Input: part model. Units: mm. Frame: model coordinates. A direction names the side the tool comes from. Give positions to 0.01 mm unless a question says otherwise; leave off trailing zeros. Loops run counter-clockwise (first coordinate to the right, second up) from the corner with the lowest first, then second, coordinate; pieces in that order, holes last. Notation, with made-up numbers: (-19.5, 82.5) -> (-13.5, 82.5) arc R22 ccw to (-13.5, 106.5) -> close; hole circle Ø7 at (56.25, 15.25). An arc over 180 degrees is marked (long way). Use CSV: the item, a comma, the result in double quotes.
```python
from build123d import *

# Parameters (mm, degrees)
SKETCH_1_R               = 3
EXTRUDE_1_DEPTH          = 180
SKETCH_2_R               = 8
EXTRUDE_2_DEPTH          = 2
EXTRUDE_START            = -178
SKETCH_2_2_R             = 8
EXTRUDE_3_DEPTH          = 2
EXTRUDE_START_2          = -2
SKETCH_1_2_R             = 3
EXTRUDE_4_DEPTH          = 2
EXTRUDE_START_3          = 180
SKETCH_1_3_R             = 3
EXTRUDE_5_DEPTH          = 2
EXTRUDE_START_4          = 4
SKETCH_2_3_R             = 8
EXTRUDE_6_DEPTH          = 2
EXTRUDE_START_5          = -182
SKETCH_2_4_R             = 8
EXTRUDE_7_DEPTH          = 2
EXTRUDE_START_6          = -64
SKETCH_3_R               = 5
EXTRUDE_10_DEPTH         = 60
CUT_EXTRUDE_1_DEPTH      = 185.347497949
CUT_EXTRUDE_1_DEPTH_BACK = 185.347497949
SKETCH_4_W               = 115.941163498
SKETCH_4_H               = 45.19740272


with BuildPart() as part:
    # 草图1 → 凸台-拉伸1 (new body)
    with BuildSketch(Plane.XY):
        with Locations(Location((0, 0, 0), (0, 0, 180))):
            Circle(SKETCH_1_R)
    extrude(amount=EXTRUDE_1_DEPTH)

    # 草图2 → 凸台-拉伸2 (add)
    with BuildSketch(Plane.XY.offset(180)):
        Circle(SKETCH_2_R)
    extrude(amount=-EXTRUDE_2_DEPTH)

    # 草图2<2> → 凸台-拉伸3 (add)
    with BuildSketch(Plane.XY.offset(180).offset(EXTRUDE_START)):
        Circle(SKETCH_2_2_R)
    extrude(amount=-EXTRUDE_3_DEPTH)

    # 草图1<2> → 凸台-拉伸4 (add)
    with BuildSketch(Plane.XY.offset(EXTRUDE_START_2)):
        with Locations(Location((0, 0, 0), (0, 0, 180))):
            Circle(SKETCH_1_2_R)
    extrude(amount=EXTRUDE_4_DEPTH)

    # 草图1<3> → 凸台-拉伸5 (add)
    with BuildSketch(Plane.XY.offset(EXTRUDE_START_3)):
        with Locations(Location((0, 0, 0), (0, 0, 180))):
            Circle(SKETCH_1_3_R)
    extrude(amount=EXTRUDE_5_DEPTH)

    # 草图2<3> → 凸台-拉伸6 (add)
    with BuildSketch(Plane.XY.offset(180).offset(EXTRUDE_START_4)):
        Circle(SKETCH_2_3_R)
    extrude(amount=-EXTRUDE_6_DEPTH)

    # 草图2<4> → 凸台-拉伸7 (add)
    with BuildSketch(Plane.XY.offset(180).offset(EXTRUDE_START_5)):
        Circle(SKETCH_2_4_R)
    extrude(amount=-EXTRUDE_7_DEPTH)

    # 草图3 → 凸台-拉伸10 (add)
    with BuildSketch(Plane.XY.offset(184).offset(EXTRUDE_START_6)):
        Circle(SKETCH_3_R)
    extrude(amount=-EXTRUDE_10_DEPTH)

    # 草图4 → 切除-拉伸1 (cut, two sides: drawn at the far end of the back side and taken through both)
    with BuildSketch(Plane(origin=(0, 0, 0), x_dir=(0, 0, -1), z_dir=(1, 0, 0)).offset(-CUT_EXTRUDE_1_DEPTH_BACK)):
        with Locations((-38.8417804, 0.262013929)):
            Rectangle(SKETCH_4_W, SKETCH_4_H)
    extrude(amount=CUT_EXTRUDE_1_DEPTH + CUT_EXTRUDE_1_DEPTH_BACK, mode=Mode.SUBTRACT)


solid = part.part
```
1) Contact query for flat-ended pins moving along their axis: pin 1 (4 mm diameter, centred on x = 0.5, z = 127.5, fed in from -Y); pin 2 (3 mm diameter, centred on x = -5.5, z = 145, fed in from -Y); pin 3 (2 mm diameter, centred on x = -1.5, z = 113, fed in from +Y); pin 4 (6 mm diameter, centred on x = 1.5, z = 122, fed in from -Y). Output: stop coordinate, or through.
From the geometry:
pin 1,"stops at y = -3"
pin 2,"passes through"
pin 3,"stops at y = 4.97"
pin 4,"stops at y = -5"
2) Section query C-C (x = -3.75). Return loops of the section in (y, z).
From the geometry:
outline,"(-7.07, 178) -> (7.07, 178) -> (7.07, 180) -> (-7.07, 180) -> close; (-7.07, 182) -> (7.07, 182) -> (7.07, 184) -> (-7.07, 184) -> close; (-3.31, 96.81) -> (3.31, 96.81) -> (3.31, 120) -> (-3.31, 120) -> close"
3) Mould query, pull axis Z, two halves, no side actions, for faces 4 (the cylindrical face through (-1.73, -7.81, 183.01)), 5 (the flat face through (0, 0, 96.812)), 6 (the flat face through (0, 0, 184)), 7 (the cylindrical face through (-2.86, -0.9, 148.59)). Classes: pulls with the +Z half, pulls with the -Z half, needs draft (parallel to the pull), parting line crosses it, or undercut.
From the geometry:
face 4,"needs draft"
face 5,"pulls with the -Z half"
face 6,"pulls with the +Z half"
face 7,"undercut"
4) Section query A-A (x = 0). Return loops of the section in (y, z).
From the geometry:
outline,"(-8, 178) -> (-3, 178) -> (-3, 120) -> (-5, 120) -> (-5, 96.81) -> (5, 96.81) -> (5, 120) -> (3, 120) -> (3, 178) -> (8, 178) -> (8, 180) -> (3, 180) -> (3, 182) -> (8, 182) -> (8, 184) -> (-8, 184) -> (-8, 182) -> (-3, 182) -> (-3, 180) -> (-8, 180) -> close"
5) Reachability of faces 1 (the cylindrical face through (-1.08, -4.88, 108.57)), 2 (the cylindrical face through (-2.86, -0.9, 180.99)), 3 (the cylindrical face through (-1.73, -7.81, 179.01)) from +Z, -Z, +X, -X, +Y, -Y: full face, straight path, thin tool, end or side. Return the list, or none.
From the geometry:
face 1,"-Z"
face 2,"none"
face 3,"+Z, -Z"
6) Section query D-D (z = 164). Return loops of the section in (x, y), then the cut area to 3 significant figures.
From the geometry:
outline,"circle Ø6 at (0, 0)"
area,"28.3 mm^2"
7) Ray query, line 1 (Z direction, x = 4.75, y = 4.25); line 2 (Z direction, x = 3.5, y = 0.25); line 3 (Y direction, x = -0.25, z = 158). Return the intervals inside material, ascending.
From the geometry:
line 1,"z = 178 to 180, 182 to 184"
line 2,"z = 96.81 to 120, 178 to 180, 182 to 184"
line 3,"y = -2.99 to 2.99"
